Part print with two shaded views. Sizes in mm from the minimum x, y, z corner. A direction names the side the tool comes from. Give positions to 0.01 mm unless a question says otherwise; leave off trailing zeros. Write each loop counter-clockwise with the first axis right and the second up, starting at its lowest first coordinate (ties: lowest second). Pieces come first, ordered by that corner, then holes. Notation, with made-up numbers: M -29.5,23.25 L -17.5,23.25 A24 cw -17.5,35.25 Z; hole C 24.25,-14 d11. An arc over 180 degrees is marked long. Return JSON: item names as keys, results as strings. Group by question number.
Q1. Wall check: probe 1 along Y at (x, z) = (2.5, 2); probe 2 along Z at (x, y) = (4.25, 2.7); probe 3 along X at (y, z) = (2.4, 10) (1 decimal). Give the ranges that are in metal, low to high.
Q2. Band-saw the part on C-C, the plane x = 3.5. Give the cut face in (y, z).
Q3. Tool access for the marked faces 1 and 2: list every direction of +Z, -Z, +X, -X, +Y, -Y with a clear straight run to the whole face (end or side of a thin tool).
Q4. Band-saw the part on B-B, the plane y = 1.05. Give the cut face in (x, z) (1 decimal).
Q5. Flat gauge pin, fed straight in: pin 1 Ø2 at (y, z) = (0.5, 3) entering from -X. Where does the tip first touch, or does it go through?
Q6. Band-saw the part on A-A, the plane z = 7.75. Give the cut face in (x, y).
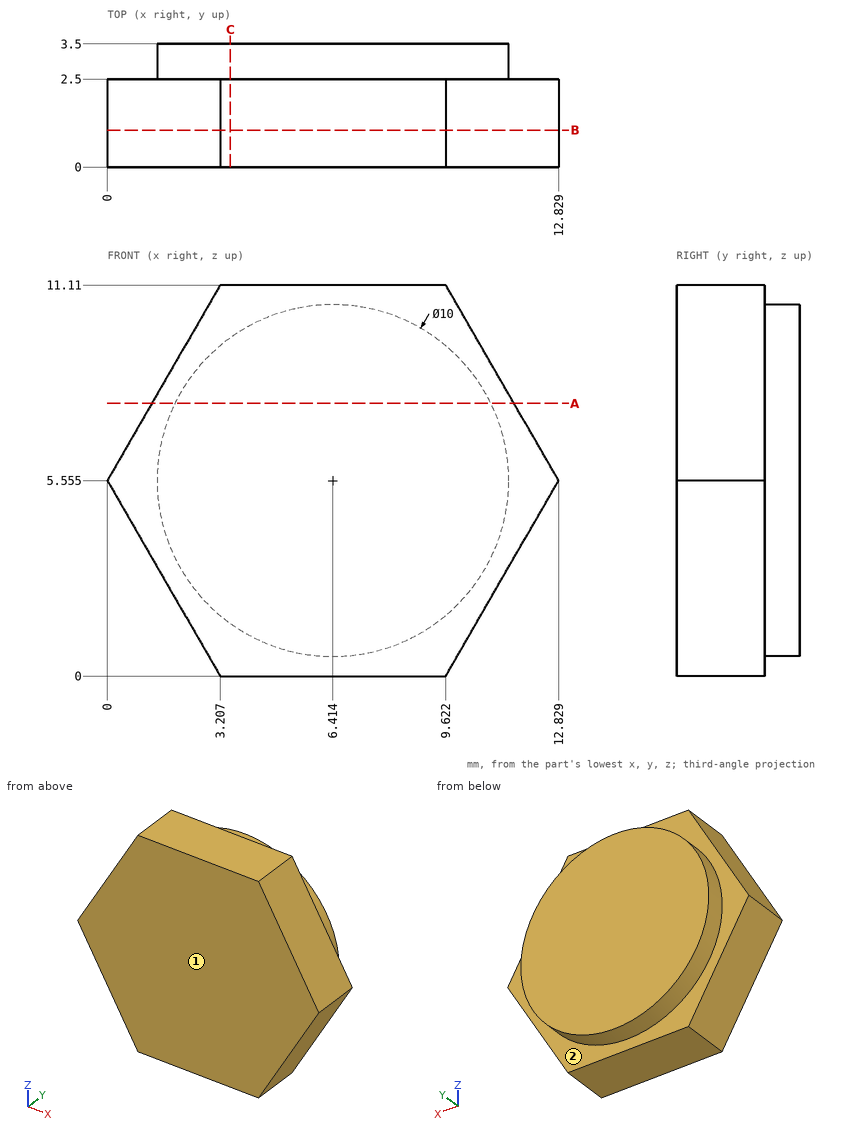
From the geometry:
{
 "1": {"probe 1": "y = 0 to 2.5", "probe 2": "z = 1.05 to 10.06", "probe 3": "x = 2.6 to 10.3"},
 "2": {"outline": "M 0,0 L 2.5,0 L 2.5,1.49 L 3.5,1.49 L 3.5,9.62 L 2.5,9.62 L 2.5,11.11 L 0,11.11 Z"},
 "3": {"face 1": "+Z, -Z, +X, -X, -Y", "face 2": "+Y"},
 "4": {"outline": "M 0,5.6 L 3.2,0 L 9.6,0 L 12.8,5.6 L 9.6,11.1 L 3.2,11.1 Z"},
 "5": {"pin 1": "stops at x = 0.9"},
 "6": {"outline": "M 1.27,0 L 11.56,0 L 11.56,2.5 L 10.91,2.5 L 10.91,3.5 L 1.92,3.5 L 1.92,2.5 L 1.27,2.5 Z"}
}
